Could you check a few things on this model? Use its own coordinates, in mm. A direction names the side the tool comes from. Coordinates: 2 decimals unless noted, no trailing zeros. Order: outer loops, then holes, each group sorted by start corner. A loop starts at its lowest first (then second) coordinate and runs counter-clockwise, first axis right, second up. Notation, with made-up numbers: (4.25, 56) - (17.25, 56) arc R11 cw to (17.25, 71) - close; hole circle Ø7 at (-24.5, 12.5). An arc over 180 degrees is marked (long way). Answer as CSV lines item,"result". Start each with the question number.
1. I want a section at A-A, the plane x = -65. List the corners of the cut face in (y, z) for me, and give its area (3 significant figures).
2. I need wall thicknesses on probe 1 along Y at (x, z) = (-65, 0.75); probe 2 along X at (y, z) = (4, 2.65); probe 3 along Y at (x, z) = (65, 1.25). Which ranges of each line are inside material? Lowest first, please.
3. For pin 1 (0.9 mm diameter, centred on x = -13, z = 1, fed in from +Y); pin 2 (0.9 mm diameter, centred on x = -10, z = 1, fed in from -Y), each with a flat end and sliding along its axis, tell me the tip position at first contact or that it passes through.
4. I want a section at B-B, the plane y = 0. List the corners of the cut face in (x, z) for me, and give its area (4 significant figures).
5. Thinking about a two-plate mould opening in Y: for faces 1 (the face through (-22, 0, 3)), 2 (the face through (-87.485, 0.812, 1.521)), 3 (the face through (-63.57, -16.55, 1.52)), which applies, released by +Y, released by -Y, zero draft, split by the parting line, or undercut?
6. I want a section at D-D, the plane z = 1.4. Count the separate pieces of the cut face and the enclosed holes in it, and give its area (3 significant figures).
7. For faces 4 (the face through (9, 12, 1)), 5 (the face through (-80.57, 0.45, 1.52)), 6 (the face through (10, -12, 1)), which set-ups out of +Z, -Z, +X, -X, +Y, -Y let a thin tool reach every point of the face, with its end or its side?
8. I want a section at C-C, the plane x = 30. List the corners of the cut face in (y, z) for me, and give its area (3 significant figures).
from build123d import *

# Parameters (mm, degrees)
BOSS_EXTRU_1_DEPTH           = 3
ESQUISSE2_R                  = 6.5
ENL_V_MAT_EXTRU_1_DEPTH      = 78.987178433
ENL_V_MAT_EXTRU_2_DEPTH      = 78.987178433
ENL_V_MAT_EXTRU_2_DEPTH_BACK = 78.987178433
ESQUISSE4_R                  = 1.5
ESQUISSE5_R                  = 22.5
ESQUISSE5_R_2                = 6.5
BOSS_EXTRU_2_DEPTH           = 3
ESQUISSE6_R                  = 1.5
ENL_V_MAT_EXTRU_3_DEPTH      = 91.396349484


with BuildPart() as part:
    # Esquisse1 → Boss.-Extru.1 (new body)
    with BuildSketch(Plane.XY):
        with BuildLine():
            Line((-65, 12), (65, 12))
            ThreePointArc((65, 12), (77, 0), (65, -12))
            Line((65, -12), (-65, -12))
            ThreePointArc((-65, -12), (-77, 0), (-65, 12))
        make_face()
    extrude(amount=BOSS_EXTRU_1_DEPTH)

    # Esquisse2 → Enlèv. mat.-Extru.1 (cut, through all)
    with BuildSketch(Plane.XY.offset(3)):
        with Locations((-65, 0)):
            Circle(ESQUISSE2_R)
        with Locations(Location((65, 0, 0), (0, 0, 180))):
            Circle(ESQUISSE2_R)
    extrude(amount=-ENL_V_MAT_EXTRU_1_DEPTH, mode=Mode.SUBTRACT)

    # Esquisse4 → Enlèv. mat.-Extru.2 (cut, two sides: drawn at the far end of the back side and taken through both)
    with BuildSketch(Plane.XY.offset(3).offset(-ENL_V_MAT_EXTRU_2_DEPTH_BACK)):
        with Locations((-30, 0)):
            Circle(ESQUISSE4_R)
        with Locations(Location((30, 0, 0), (0, 0, 180))):
            Circle(ESQUISSE4_R)
    extrude(amount=ENL_V_MAT_EXTRU_2_DEPTH + ENL_V_MAT_EXTRU_2_DEPTH_BACK, mode=Mode.SUBTRACT)

    # Esquisse5 → Boss.-Extru.2 (add)
    with BuildSketch(Plane.XY.offset(3)):
        with Locations((-65, 0)):
            Circle(ESQUISSE5_R)
        with Locations((-65, 0)):
            Circle(ESQUISSE5_R_2, mode=Mode.SUBTRACT)
    extrude(amount=-BOSS_EXTRU_2_DEPTH)

    # Esquisse6 → Enlèv. mat.-Extru.3 (cut, through all)
    with BuildSketch(Plane.XY.offset(3)):
        with Locations((-65, 17)):
            Circle(ESQUISSE6_R)
        with Locations((-48, 0)):
            Circle(ESQUISSE6_R)
        with Locations((-65, -17)):
            Circle(ESQUISSE6_R)
        with Locations((-82, 0)):
            Circle(ESQUISSE6_R)
    extrude(amount=-ENL_V_MAT_EXTRU_3_DEPTH, mode=Mode.SUBTRACT)


solid = part.part
Solved:
1,outline,"(-22.5, 0) - (-18.5, 0) - (-18.5, 3) - (-22.5, 3) - close; (-15.5, 0) - (-6.5, 0) - (-6.5, 3) - (-15.5, 3) - close; (6.5, 0) - (15.5, 0) - (15.5, 3) - (6.5, 3) - close; (18.5, 0) - (22.5, 0) - (22.5, 3) - (18.5, 3) - close"
1,area,"78.0 mm2"
2,probe 1,"y = -22.5 to -18.5, -15.5 to -6.5, 6.5 to 15.5, 18.5 to 22.5"
2,probe 2,"x = -87.14 to -70.12, -59.88 to 59.88, 70.12 to 76.31"
2,probe 3,"y = -12 to -6.5, 6.5 to 12"
3,pin 1,"stops at y = 12"
3,pin 2,"stops at y = -12"
4,outline,"(-87.5, 0) - (-83.5, 0) - (-83.5, 3) - (-87.5, 3) - close; (-80.5, 0) - (-71.5, 0) - (-71.5, 3) - (-80.5, 3) - close; (-58.5, 0) - (-49.5, 0) - (-49.5, 3) - (-58.5, 3) - close; (-46.5, 0) - (-31.5, 0) - (-31.5, 3) - (-46.5, 3) - close; (-28.5, 0) - (28.5, 0) - (28.5, 3) - (-28.5, 3) - close; (31.5, 0) - (58.5, 0) - (58.5, 3) - (31.5, 3) - close; (71.5, 0) - (77, 0) - (77, 3) - (71.5, 3) - close"
4,area,"379.5 mm2"
5,face 1,"zero draft"
5,face 2,"split by the parting line"
5,face 3,"undercut"
6,separate pieces,"1"
6,enclosed holes,"8"
6,area,"4,120 mm2"
7,face 4,"+Z, -Z, +X, +Y"
7,face 5,"+Z, -Z"
7,face 6,"+Z, -Z, +X, -Y"
8,outline,"(-12, 0) - (-1.5, 0) - (-1.5, 3) - (-12, 3) - close; (1.5, 0) - (12, 0) - (12, 3) - (1.5, 3) - close"
8,area,"63.0 mm2"
